Can you work these out from the model? Positions are in its coordinate system, mm. A direction names the side the tool comes from. Coordinates: 2 decimals unless noted, no trailing zeros. Loops run counter-clockwise (first coordinate to the right, second up) from the corner with the lowest first, then second, coordinate; pieces in that order, holes last.
Solid Edge part; units mm, degrees
sketch "Sketch1" plane through (0, 0, 0) normal (0, 0, 1) x (1, 0, 0)
  circle A0 centre (45, -22.5) radius 10
  arc A1 (-45, 0) -> (-45, -45) centre (-45, -22.5) ccw
  line L0 (-45, -45) -> (45, -45)
  arc A2 (45, -45) -> (45, 0) centre (45, -22.5) ccw
  line L1 (0, 0) -> (45, 0)
  line L2 (0, 0) -> (-45, 0)
  circle A3 centre (-45, -22.5) radius 10
extrude "Protrusion1" add sketch "Sketch1" against normal blind 15
sketch "Sketch2" plane through (0, 0, 71.6) normal (0, 0, 1) x (1, 0, 0)
  line L0 (15, -30) -> (15, 0)
  line L1 (15, 0) -> (-15, 0)
  line L2 (-15, 0) -> (-15, -30)
  line L3 (-15, -30) -> (15, -30)
extrude "ExtrudedProtrusion_2" add sketch "Sketch2" along normal mid plane 30
sketch "Sketch3" plane through (0, -30, 71.6) normal (0, -1, 0) x (1, 0, 0)
  line L0 (10, -10) -> (10, 10)
  line L1 (10, 10) -> (-10, 10)
  line L2 (-10, 10) -> (-10, -10)
  line L3 (-10, -10) -> (10, -10)
extrude "ExtrudedCutout_1" cut sketch "Sketch3" against normal blind 30
sketch "Sketch4" plane through (0, -15, 71.6) normal (0, -1, 0) x (1, 0, 0)
  line L0 (15, 12) -> (40, 12)
  arc A0 (40, 12) -> (40, -12) centre (40, 0) cw
  line L1 (40, -12) -> (15, -12)
  line L2 (15, 12) -> (15, -12)
  circle A1 centre (40, 0) radius 5
extrude "ExtrudedProtrusion_3" add sketch "Sketch4" along normal mid plane 10
sketch "Sketch5" plane through (0, -15, 71.6) normal (0, -1, 0) x (1, 0, 0)
  line L0 (-15, 12) -> (-15, -12)
  line L1 (-40, -12) -> (-15, -12)
  arc A0 (-40, 12) -> (-40, -12) centre (-40, 0) ccw
  line L2 (-15, 12) -> (-40, 12)
  circle A1 centre (-40, 0) radius 5
extrude "ExtrudedProtrusion_4" add sketch "Sketch5" along normal mid plane 10
sketch "Sketch6" plane through (0, 0, 0) normal (1, 0, 0) x (0, 1, 0)
  line L0 (-30, 56.6) -> (-22.5, 56.6)
  line L1 (-22.5, 0) -> (-22.5, 56.6)
  line L2 (-45, 0) -> (-22.5, 0)
  line L3 (-30, 56.6) -> (-45, 0)
extrude "ExtrudedProtrusion_5" add sketch "Sketch6" along normal mid plane 15
sketch "Sketch7" plane through (0, -22.5, 0) normal (0, -1, 0) x (1, 0, 0)
  line L0 (24.5, 0) -> (15, 56.6)
  line L1 (-15, 56.6) -> (15, 56.6)
  line L2 (-24.5, 0) -> (-15, 56.6)
  line L3 (0, 0) -> (-24.5, 0)
  line L4 (0, 0) -> (24.5, 0)
extrude "ExtrudedProtrusion_6" add sketch "Sketch7" against normal blind 22.5
fillet "Round_1" radius 3 4 edges at (15, -15, 83.6) (-15, -15, 83.6) (15, -15, 59.6) (-15, -15, 59.6)
(1) I want a section at B-B on z = 71.6. Write out the boundary of the cut face in (x, y), then the cut area to 3 significant figures.
Check values:
outline: (-52, -20) - (-45, -20) - (-45, -10) - (-52, -10) - close; (-35, -20) - (-15, -20) - (-15, -30) - (-10, -30) - (-10, 0) - (-15, 0) - (-15, -10) - (-35, -10) - close; (10, -30) - (15, -30) - (15, -20) - (35, -20) - (35, -10) - (15, -10) - (15, 0) - (10, 0) - close; (45, -20) - (52, -20) - (52, -10) - (45, -10) - close
area: 840 mm2
(2) I want a section at D-D on y = -41. Write out the boundary of the cut face in (x, z), then the cut area to 3 significant figures.
Check values:
outline: (-57.81, -15) - (57.81, -15) - (57.81, 0) - (7.5, 0) - (7.5, 15.09) - (-7.5, 15.09) - (-7.5, 0) - (-57.81, 0) - close
area: 1,960 mm2
(3) If we mould it in two halves opening along X, with no side actions, what happens to faces 5 (the flat face through (-15, -21, 71)), 6 (the flat face through (10, -15, 71)), 7 (the cylindrical face through (15.9, -15.07, 58.74))? For each: released by +X, released by -X, zero draft, split by the parting line, or undercut.
Check values:
face 5: released by -X
face 6: undercut
face 7: released by +X
(4) I want a section at A-A on x = -32.5. Write out the boundary of the cut face in (y, z), then the cut area to 3 significant figures.
Check values:
outline: (-45, -15) - (0, -15) - (0, 0) - (-45, 0) - close; (-20, 59.6) - (-10, 59.6) - (-10, 83.6) - (-20, 83.6) - close
area: 915 mm2
(5) I'm going to push flat-ended pins straight in: pin 1 (13.5 mm diameter, centred on x = 20, z = 33.5, fed in from -Y); pin 2 (24 mm diameter, centred on x = -32.5, z = 79, fed in from -Y); pin 3 (11.5 mm diameter, centred on x = -40, z = 71.6, fed in from +Y); pin 4 (6 mm diameter, centred on x = 10.5, z = 19.5, fed in from +Y). Where does each tip first touch, or does it pass through?
Check values:
pin 1: stops at y = -22.5
pin 2: stops at y = -20
pin 3: stops at y = -10
pin 4: stops at y = 0
(6) If I drill on probe 1 along Z at (x, y) = (40, -13.25); probe 2 along Y at (x, z) = (-45, -11.25); probe 3 along Z at (x, y) = (-40, -17), over which ranges is the centre line in solid material (lowest first)?
Check values:
probe 1: z = -15 to 0, 59.6 to 66.6, 76.6 to 83.6
probe 2: y = -45 to -32.5, -12.5 to 0
probe 3: z = 59.6 to 66.6, 76.6 to 83.6
(7) Which directions (+Z, -Z, +X, -X, +Y, -Y) give clear straight access to the entire face, cutting with the end or side of a thin tool? Please do faces 1 (the flat face through (29, -15, 59.6)), 2 (the flat face through (-14, -22.5, 22)), 3 (the cylindrical face through (-15.9, -14.93, 58.74)), 4 (the flat face through (0, -15, 81.6)).
Check values:
face 1: +X, +Y, -Y
face 2: -X, -Y
face 3: -X, +Y, -Y
face 4: +Y, -Y
(8) I want a section at C-C on x = 50. Write out the boundary of the cut face in (y, z).
Check values:
outline: (-44.44, -15) - (-31.16, -15) - (-31.16, 0) - (-44.44, 0) - close; (-20, 64.97) - (-10, 64.97) - (-10, 78.23) - (-20, 78.23) - close; (-13.84, -15) - (-0.56, -15) - (-0.56, 0) - (-13.84, 0) - close
